from build123d import *

# Parameters (mm, degrees)
PAD_DEPTH         = 22
SKETCH001_R       = 3.1
POCKET_DEPTH      = 5.001
POCKET_DEPTH_BACK = -27.001
SKETCH002_R       = 3.1
POCKET001_DEPTH   = 5
SKETCH003_R       = 1.6
POCKET002_DEPTH   = 44.001
FILLET_R          = 2
SKETCH004_R       = 1.95
POCKET003_DEPTH   = 8


with BuildPart() as part:
    # Sketch → Pad (new body, symmetric)
    with BuildSketch(Plane.XZ):
        Polygon((0, 27), (0, 0), (27, 0), (27, -5), (-32, -5), (-32, 7), (-5, 7), (-5, 27), align=None)
    extrude(amount=PAD_DEPTH, both=True)

    # Sketch001 → Pocket (cut, two sides)
    with BuildSketch(Plane.XY) as pocket_sk:
        with Locations((15, 12.5)):
            Circle(SKETCH001_R)
        with Locations((15, -12.5)):
            Circle(SKETCH001_R)
        with BuildLine():
            ThreePointArc((-16.803848, -3), (-26.859933, 3.518672), (-17.527864, -4))
            Line((-6, -4), (-17.527864, -4))
            Line((-6, -4), (-6, -10))
            Line((-6, -10), (-22, -10))
            ThreePointArc((-29.660444, 6.427876), (-31.063078, -4.226183), (-22, -10))
            Line((-18.392302, 19.856726), (-29.660444, 6.427876))
            ThreePointArc((-13.796055, 22), (-16.331753, 21.437843), (-18.392302, 19.856726))
            Line((-13.796055, 22), (-13.796055, 28.799225))
            Line((-13.796055, 28.799225), (-40.339119, 28.799225))
            Line((-40.339119, 28.799225), (-40.339119, -28.958258))
            Line((-40.339119, -28.958258), (-5, -28.958258))
            Line((-5, -28.958258), (-5, -3))
            Line((-16.803848, -3), (-5, -3))
        make_face()
    extrude(amount=-POCKET_DEPTH, mode=Mode.SUBTRACT)
    extrude(pocket_sk.sketch, amount=-POCKET_DEPTH_BACK, mode=Mode.SUBTRACT)

    # Sketch002 → Pocket001 (cut)
    with BuildSketch(Plane.YZ):
        with Locations((-12.5, 15)):
            Circle(SKETCH002_R)
        with Locations((12.5, 15)):
            Circle(SKETCH002_R)
    extrude(amount=-POCKET001_DEPTH, mode=Mode.SUBTRACT)

    # Sketch003 (on Face5 of Pocket001) → Pocket002 (cut, through all)
    with BuildSketch(Plane(origin=(0, 22, 0), x_dir=(1, 0, 0), z_dir=(0, 1, 0))):
        with Locations((-11, -1)):
            Circle(SKETCH003_R)
    extrude(amount=-POCKET002_DEPTH, mode=Mode.SUBTRACT)

    # Fillet
    fillet_edges = [part.edges().sort_by_distance(p)[0] for p in [
        (-6, -4, 1),
        (-6, -10, 1),
        (-5, -3, 1),
        (-5, 9.5, 7),
        (27, -22, -2.5),
        (27, 22, -2.5),
        (0, 0, 0),
        (-2.5, -22, 27),
        (-2.5, 22, 27),
    ]]
    fillet(fillet_edges, radius=FILLET_R)

    # Sketch004 (on Face2 of Fillet) → Pocket003 (cut)
    with BuildSketch(Plane(origin=(0, 22, 0), x_dir=(1, 0, 0), z_dir=(0, 1, 0))):
        with Locations((-11, -1)):
            Circle(SKETCH004_R)
    extrude(amount=-POCKET003_DEPTH, mode=Mode.SUBTRACT)


solid = part.part
Build history of the part. All positions in model axes, mm. A direction names the side the tool comes from. Coordinates: 2 decimals unless noted, no trailing zeros. Order: outer loops, then holes, each group sorted by start corner. A loop starts at its lowest first (then second) coordinate and runs counter-clockwise, first axis right, second up. Notation, with made-up numbers: (-28, 73.25) -> (-22, 73.25) arc R18 cw to (-22, 99.25) -> close; hole circle Ø9 at (28.5, -31). An arc over 180 degrees is marked (long way). One line per item, written item: value.
(1) Slice it at B-B, the plane x = 15. List the corners of the cut face in (y, z).
Checked values:
outline: (-22, -5) -> (-15.6, -5) -> (-15.6, 0) -> (-22, 0) -> close; (-9.4, -5) -> (9.4, -5) -> (9.4, 0) -> (-9.4, 0) -> close; (15.6, -5) -> (22, -5) -> (22, 0) -> (15.6, 0) -> close
(2) Slice it at C-C, the plane z = 15. List the corners of the cut face in (x, y).
Checked values:
outline: (-5, -22) -> (0, -22) -> (0, -15.6) -> (-5, -15.6) -> close; (-5, -9.4) -> (0, -9.4) -> (0, 9.4) -> (-5, 9.4) -> close; (-5, 15.6) -> (0, 15.6) -> (0, 22) -> (-5, 22) -> close
(3) Drop flat-ended pins along their axis: pin 1 Ø5 at (y, z) = (12.5, 15) entering from +X; pin 2 Ø10 at (y, z) = (-12.5, 15) entering from +X; pin 3 Ø0.6 at (y, z) = (-7.5, 1.5) entering from +X; pin 4 Ø1.5 at (y, z) = (-9, 23) entering from -X. Give the stop position or say it passes through.
Checked values:
pin 1: through
pin 2: x = 0
pin 3: x = 0.17
pin 4: x = -5
(4) Mould opens along Z. For faces 1 (the cylindrical face through (-9.14, 18.06, 0.41)), 2 (the cylindrical face through (-6.57, -9.4, 1.08)), 3 (the flat face through (4, 0, -5)) say: pulls with the +Z half, pulls with the -Z half, needs draft (parallel to the pull), parting line crosses it, or undercut.
Checked values:
face 1: undercut
face 2: needs draft
face 3: pulls with the -Z half
(5) Tool access for faces 4 (the flat face through (-13, -3, 1)), 5 (the cylindrical face through (26.4, -21.43, -2.54)), 6 (the flat face through (-6, -7, 1)): list every direction of +Z, -Z, +X, -X, +Y, -Y with a clear straight run to the whole face (end or side of a thin tool).
Checked values:
face 4: +Z, -Z
face 5: +Z, -Z, +X, -Y
face 6: +Z, -Z, -Y
(6) Probe line 1 (X direction, y = -6.6, z = 1); line 2 (Z direction, x = -11, y = -5.2); line 3 (Y direction, x = -8, z = 2). List the from-to ranges inside material, lowest first. Write a range as [from, to].
Checked values:
line 1: [-29.51, -12.6], [-9.4, -6], [-5, 0.27]
line 2: [-5, -0.6], [2.6, 7]
line 3: [-10, -4], [-3, 22]
(7) Slice it at D-D, the plane y = 12.5. List the corners of the cut face in (x, z), plus the area to 3 significant figures.
Checked values:
outline: (-24.57, -5) -> (11.9, -5) -> (11.9, 0) -> (2, 0) arc R2 cw to (0, 2) -> (0, 11.9) -> (-5, 11.9) -> (-5, 9) arc R2 cw to (-7, 7) -> (-24.57, 7) -> close; (-5, 18.1) -> (0, 18.1) -> (0, 27) -> (-5, 27) -> close; (18.1, -5) -> (27, -5) -> (27, 0) -> (18.1, 0) -> close; hole circle Ø3.2 at (-11, 1)
area: 461 mm2
(8) Slice it at A-A, the plane y = -1. List the corners of the cut face in (x, z), plus the area to 3 significant figures.
Checked values:
outline: (-31.95, -5) -> (-27.92, -5) -> (-27.92, 7) -> (-31.95, 7) -> close; (-16.08, -5) -> (27, -5) -> (27, 0) -> (2, 0) arc R2 cw to (0, 2) -> (0, 27) -> (-5, 27) -> (-5, 9) arc R2 cw to (-7, 7) -> (-16.08, 7) -> close; hole circle Ø3.2 at (-11, 1)
area: 470 mm2
